Design review of the part shown in the three views and the two pictorial views. Dimensions are in mm from the part's minimum x, y and z. A direction names the side the tool comes from. Coordinates: 2 decimals unless noted, no trailing zeros. Order: outer loops, then holes, each group sorted by start corner. A loop starts at its lowest first (then second) coordinate and runs counter-clockwise, first axis right, second up. Notation, with made-up numbers: (-35.5, 18) -> (-23.5, 18) arc R20 cw to (-23.5, 50) -> close; hole circle Ø7 at (-5, 36). An arc over 180 degrees is marked (long way). Answer as a JSON object with one key per item and string values. Group by question number.
1) For pin 1 (5 mm diameter, centred on y = 10.5, z = 22.5, fed in from +X); pin 2 (3.5 mm diameter, centred on x = 10, y = 13, fed in from +Z); pin 3 (3.5 mm diameter, centred on x = 9, y = 16, fed in from -Z), all flat-tipped, find the tip position at first contact; note any pin that passes through.
2) Add section A-A, the plane y = 5. Write out the cut boundary in (x, z).
3) Add section C-C, the plane x = 11. Write out the cut boundary in (y, z), then the cut area to 3 significant figures.
4) Machinability: for the marked faces 1, 2, 3 and 4, which of the approach directions +Z, -Z, +X, -X, +Y, -Y give a long, thin tool a straight path to every point of the face, cutting with its end or side? Answer none if there is none.
5) Add section D-D, the plane y = 37. Write out the cut boundary in (x, z), then the cut area to 3 significant figures.
6) Wall thickness on L1, parallel to Z at x = 13, y = 16; L2, parallel to Z at x = 11, y = 38; L3, parallel to Y at x = 8.25, z = 3.25: over which ranges is each line inside the solid? List them lowest first.
7) Add section B-B, the plane z = 24. Write out the cut boundary in (x, y).
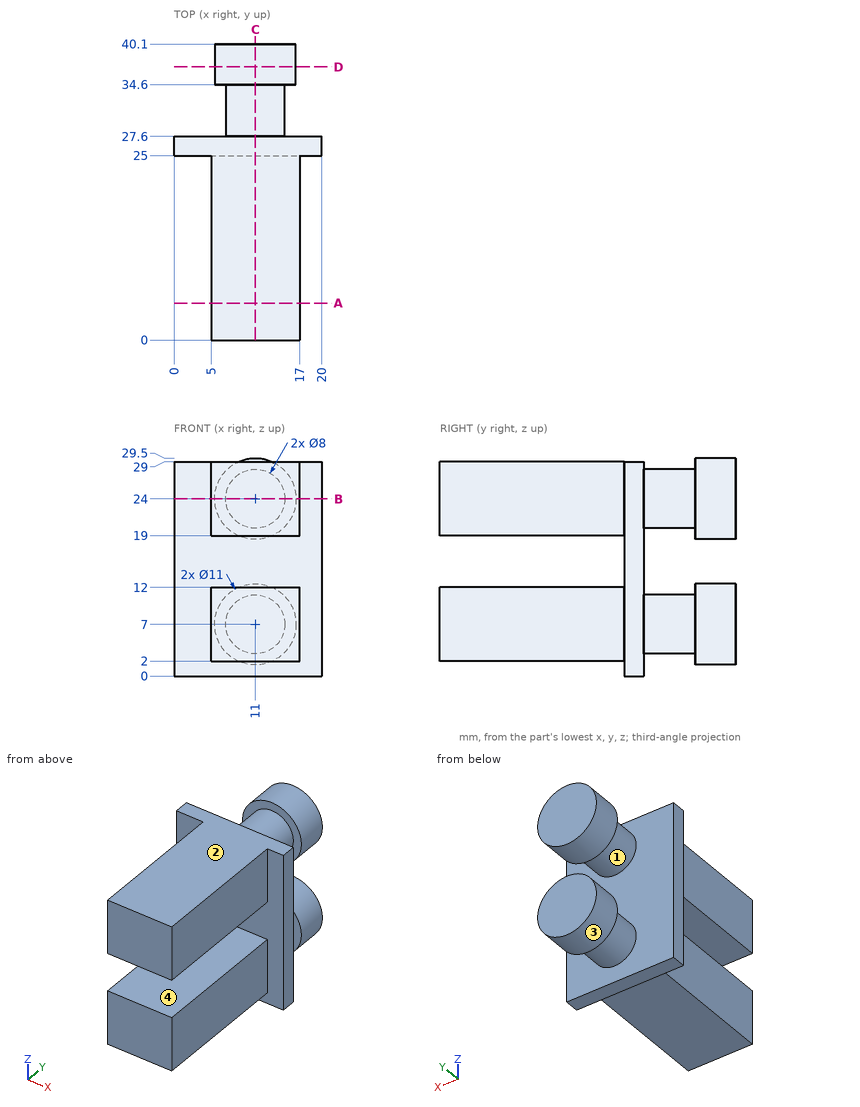
Output values:
{
 "1": {"pin 1": "stops at x = 17", "pin 2": "stops at z = 29", "pin 3": "stops at z = 2"},
 "2": {"outline": "(5, 2) -> (17, 2) -> (17, 12) -> (5, 12) -> close; (5, 19) -> (17, 19) -> (17, 29) -> (5, 29) -> close"},
 "3": {"outline": "(0, 2) -> (25, 2) -> (25, 0) -> (27.6, 0) -> (27.6, 3) -> (34.6, 3) -> (34.6, 1.5) -> (40.1, 1.5) -> (40.1, 12.5) -> (34.6, 12.5) -> (34.6, 11) -> (27.6, 11) -> (27.6, 20) -> (34.6, 20) -> (34.6, 18.5) -> (40.1, 18.5) -> (40.1, 29.5) -> (34.6, 29.5) -> (34.6, 28) -> (27.6, 28) -> (27.6, 29) -> (0, 29) -> (0, 19) -> (25, 19) -> (25, 12) -> (0, 12) -> close", "area": "808 mm²"},
 "4": {"face 1": "none", "face 2": "+Z, +X, -X, -Y", "face 3": "+Y", "face 4": "+X, -X, -Y"},
 "5": {"outline": "circle Ø11 at (11, 7); circle Ø11 at (11, 24)", "area": "190 mm²"},
 "6": {"L1": "z = 2 to 12, 19 to 29", "L2": "z = 1.5 to 12.5, 18.5 to 29.5", "L3": "y = 0 to 27.6, 34.6 to 40.1"},
 "7": {"outline": "(0, 25) -> (5, 25) -> (5, 0) -> (17, 0) -> (17, 25) -> (20, 25) -> (20, 27.6) -> (15, 27.6) -> (15, 34.6) -> (16.5, 34.6) -> (16.5, 40.1) -> (5.5, 40.1) -> (5.5, 34.6) -> (7, 34.6) -> (7, 27.6) -> (0, 27.6) -> close"}
}
